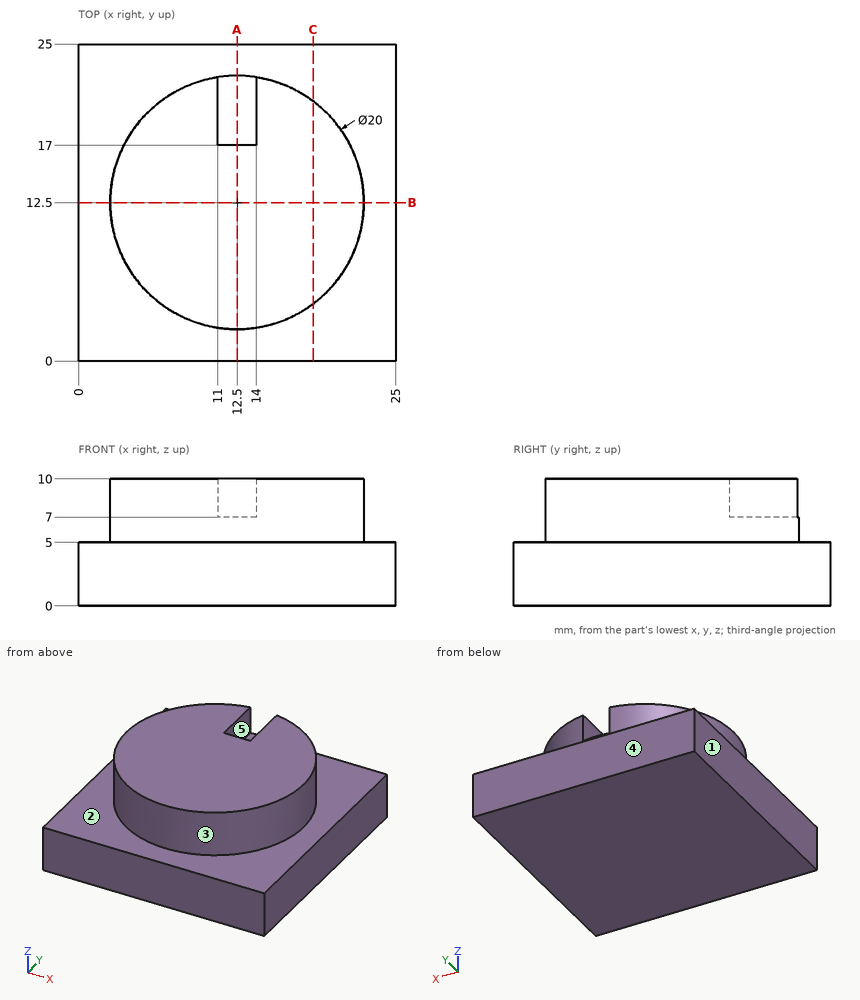
Answer from the drawing. Dimensions are ordinates in mm from the lowest x, y and z of the part. A direction names the side the tool comes from. Give positions to 0.01 mm unless a question says otherwise; leave off trailing zeros. Write each loop counter-clockwise with the first axis right and the second up, starting at its lowest first coordinate (ties: lowest second). Pieces come first, ordered by that corner, then holes. Notation, with made-up numbers: (43, 38) - (49, 38) arc R12 ccw to (49, 49) - close; hole circle Ø9 at (74.25, -25). An arc over 180 degrees is marked (long way). Answer in a Markdown table with one row per item. Add a question column.
Item 1: A tool of negligible diameter and unlimited length cuts with its end or side. For the marked faces 1 and 2, from which of +Z, -Z, +X, -X, +Y, -Y can it reach the whole face along a straight path? Write none if from no direction.
Item 2: Section C-C, the plane x = 18.5 is taken. Write down the section's boundary in (y, z).
Item 3: Section A-A, the plane x = 12.5 is taken. Write down the section's boundary in (y, z).
Item 4: Find the intervals of material crossed by L1, parallel to Z at x = 7.75, y = 2.5; L2, parallel to Z at x = 12.5, y = 19.25; L3, parallel to X at y = 17.5, z = 7.5, in increasing order.
Item 5: Section B-B, the plane y = 12.5 is taken. Write down the section's boundary in (x, z), and give its area (3 significant figures).
Item 6: Flat-ended cylindrical pins translate along their axes: P1, Ø3.5, axis at x = 12.5, y = 19.5, coming from the +Z side; P2, Ø3.5, axis at y = 20.5, z = 8, coming from the +X side; P3, Ø1.5, axis at x = 8.5, z = 8.5, coming from the -Y side; P4, Ø3, axis at x = 14.5, z = 8, coming from the +Y side. Find the tip coordinate at first contact, or state that the pin passes through.
Item 7: Determine the mould class of the marked faces 3, 4 and 5 for opening direction X: pulls with the +X half, pulls with the -X half, needs draft (parallel to the pull), parting line crosses it, or undercut.
Recorded:
| question | item | result |
|---|---|---|
| 1 | face 1 | +Z, -Z, -X, +Y, -Y |
| 1 | face 2 | +Z |
| 2 | outline | (0, 0) - (25, 0) - (25, 5) - (20.5, 5) - (20.5, 10) - (4.5, 10) - (4.5, 5) - (0, 5) - close |
| 3 | outline | (0, 0) - (25, 0) - (25, 5) - (22.5, 5) - (22.5, 7) - (17, 7) - (17, 10) - (2.5, 10) - (2.5, 5) - (0, 5) - close |
| 4 | L1 | z = 0 to 5 |
| 4 | L2 | z = 0 to 7 |
| 4 | L3 | x = 3.84 to 11, 14 to 21.16 |
| 5 | outline | (0, 0) - (25, 0) - (25, 5) - (22.5, 5) - (22.5, 10) - (2.5, 10) - (2.5, 5) - (0, 5) - close |
| 5 | area | 225 mm2 |
| 6 | P1 | stops at z = 10 |
| 6 | P2 | stops at x = 20.31 |
| 6 | P3 | stops at y = 3.04 |
| 6 | P4 | stops at y = 22.46 |
| 7 | face 3 | parting line crosses it |
| 7 | face 4 | needs draft |
| 7 | face 5 | undercut |
